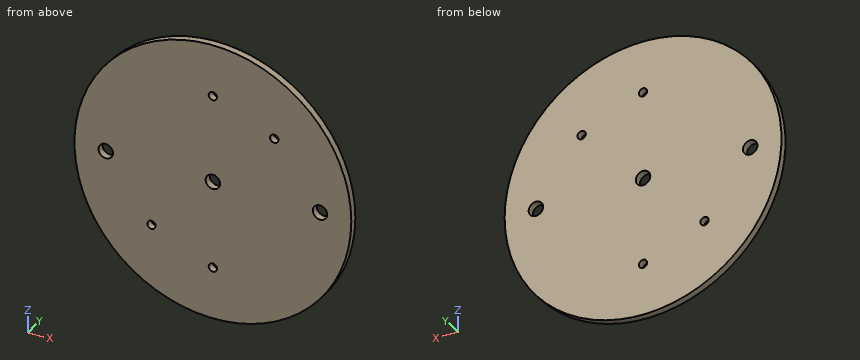
from build123d import *

# Parameters (mm, degrees)
SKETCH2_R           = 60.706
SKETCH2_R_2         = 3.175
SKETCH2_R_3         = 1.8288
BOSS_EXTRUDE1_DEPTH = 3.175


with BuildPart() as part:
    # Sketch2 → Boss-Extrude1 (new body)
    with BuildSketch(Plane(origin=(0, 0, 0), x_dir=(1, 0, 0), z_dir=(0, 1, 0))):
        Circle(SKETCH2_R)
        with Locations((-46.99, 0)):
            Circle(SKETCH2_R_2, mode=Mode.SUBTRACT)
        with Locations((46.99, 0)):
            Circle(SKETCH2_R_2, mode=Mode.SUBTRACT)
        Circle(SKETCH2_R_2, mode=Mode.SUBTRACT)
        with Locations((0, 38.1)):
            Circle(SKETCH2_R_3, mode=Mode.SUBTRACT)
        with Locations((0, -38.1)):
            Circle(SKETCH2_R_3, mode=Mode.SUBTRACT)
        with Locations((-26.940768363, 26.940768363)):
            Circle(SKETCH2_R_3, mode=Mode.SUBTRACT)
        with Locations((26.940768363, -26.940768363)):
            Circle(SKETCH2_R_3, mode=Mode.SUBTRACT)
    extrude(amount=BOSS_EXTRUDE1_DEPTH)


solid = part.part
Build history of the part. All positions in model axes, mm. Coordinates: 2 decimals unless noted, no trailing zeros. Order: outer loops, then holes, each group sorted by start corner. A loop starts at its lowest first (then second) coordinate and runs counter-clockwise, first axis right, second up. Notation, with made-up numbers: (39, 59) - (74, 59) arc R26 cw to (74, 98) - close; hole circle Ø6 at (51.5, 49.25). An arc over 180 degrees is marked (long way). Write each question's results on one line, items separated by ' | '. Start each with the question number.
Item 1: Band-saw the part on B-B on y = 1.45. Write the cut outline in (x, z) (3 decimals).
Item 2: Wall check: probe 1 along Z at (x, y) = (0, 1.2) (3 decimals); probe 2 along X at (y, z) = (0.9, 0) (3 decimals); probe 3 along Z at (x, y) = (-0.5, 1.4). Give the ranges that are in metal, low to high. Write a range as [from, to].
Item 3: Band-saw the part on D-D on x = -46.99. Write the cut outline in (y, z) (3 decimals), and give its area (3 significant figures).
Item 4: Flat gauge pins, fed straight in: pin 1 (5 mm diameter, centred on x = -26, z = -34, fed in from -Y); pin 2 (1 mm diameter, centred on x = 28.5, y = 0.5, fed in from +Z). Where does each tip first touch, or does it go through?
Item 5: Band-saw the part on A-A on x = 0. Write the cut outline in (y, z) (3 decimals).
Item 6: Band-saw the part on C-C on z = -38.1. Write the cut outline in (x, y) (3 decimals).
Numbers:
1) outline: circle Ø121.412 at (0, 0); hole circle Ø6.35 at (-46.99, 0); hole circle Ø3.658 at (-26.941, -26.941); hole circle Ø6.35 at (0, 0); hole circle Ø3.658 at (0, -38.1); hole circle Ø3.658 at (0, 38.1); hole circle Ø3.658 at (26.941, 26.941); hole circle Ø6.35 at (46.99, 0)
2) probe 1: [-60.706, -39.929], [-36.271, -3.175], [3.175, 36.271], [39.929, 60.706] | probe 2: [-60.706, -50.165], [-43.815, -3.175], [3.175, 43.815], [50.165, 60.706] | probe 3: [-60.7, -39.86], [-36.34, -3.14], [3.14, 36.34], [39.86, 60.7]
3) outline: (0, -38.434) - (3.175, -38.434) - (3.175, -3.175) - (0, -3.175) - close; (0, 3.175) - (3.175, 3.175) - (3.175, 38.434) - (0, 38.434) - close | area: 224 mm^2
4) pin 1: y = 0 | pin 2: z = 53.86
5) outline: (0, -60.706) - (3.175, -60.706) - (3.175, -39.929) - (0, -39.929) - close; (0, -36.271) - (3.175, -36.271) - (3.175, -3.175) - (0, -3.175) - close; (0, 3.175) - (3.175, 3.175) - (3.175, 36.271) - (0, 36.271) - close; (0, 39.929) - (3.175, 39.929) - (3.175, 60.706) - (0, 60.706) - close
6) outline: (-47.261, 0) - (-1.829, 0) - (-1.829, 3.175) - (-47.261, 3.175) - close; (1.829, 0) - (47.261, 0) - (47.261, 3.175) - (1.829, 3.175) - close
